Geometry check sheet. Reference: the model listing, model coordinates, mm. A direction names the side the tool comes from. Round coordinates to 2 decimals unless told otherwise and drop trailing zeros. Write each loop counter-clockwise with the first axis right and the second up, starting at its lowest first coordinate (ties: lowest second). Pieces come first, ordered by that corner, then holes. Notation, with made-up numbers: (-18.75, -27.5) -> (37.25, -27.5) arc R27 cw to (37.25, -10.5) -> close; hole circle Ø2 at (61, -2.5). An arc over 180 degrees is marked (long way). Return JSON: item names as keys, results as strings. Group by question number.
from build123d import *


with BuildPart() as f1:
    # F0 (on Front) → F1 (revolve)
    with BuildSketch(Plane.XZ):
        Polygon((0, -62), (0, 0), (-8, 0), (-8, -3.5), (-6, -3.5), (-6, -9.3), (-8, -9.3), (-8, -12.3), (-5.087018, -12.3), (-5.087018, -47.38391), (-6.285568, -47.38391), (-6.285568, -47.808396), (-5.087018, -47.808396), (-5.087018, -48.432641), (-9.75637, -48.432641), (-9.75637, -49.056886), (-5.087018, -49.056886), (-5.087018, -49.731071), (-9.75637, -49.731071), (-9.75637, -50.480166), (-5.087018, -50.480166), (-5.087018, -62), align=None)
    revolve(axis=Axis((0, 0, -31), (0, 0, 1)))


solid = f1.part
1) Go/stop test with flat-tipped pins: P1, Ø8, axis at y = 5.5, z = -50.5, coming from the +X side; P2, Ø1.5, axis at y = 1, z = -22.5, coming from the +X side; P3, Ø3, axis at x = -7.5, z = -12.5, coming from the -Y side. Record where each tip stops, or that it passes through.
2) Sectioned sample at A-A on z = -53.5. Enter the section's corners in (x, y).
3) Material ranges on probe 1 along Z at (x, y) = (-2.75, -5); probe 2 along Z at (x, y) = (-5.75, 3.75); probe 3 along Z at (x, y) = (4, -8.25), recorded low to high. Write a range as [from, to].
4) Tool access check on faces 1 (the face through (0.662, -5.044, -30.088)), 2 (the face through (1.73, 7.81, -1.77)), 3 (the face through (0.662, -5.044, -56.321)). Record the directions out of +Z, -Z, +X, -X, +Y, -Y that give a thin tool (end or side, any length) a straight path to the whole face; none if there is none.
5) Mould release check, pull along Z, two halves, no side actions. Record for faces 4 (the face through (-2, 5, -47.808)), 5 (the face through (1.27, -9.673, -48.749)), 6 (the face through (-4, 4, -50.48)), 7 (the face through (2, -6, -3.5)): +Z half, -Z half, draft (parallel to the pull), parting line (faces both ways), or undercut.
Evaluation:
{
 "1": {"P1": "stops at x = 9.64", "P2": "stops at x = 5.08", "P3": "stops at y = -5.28"},
 "2": {"outline": "circle Ø10.17 at (0, 0)"},
 "3": {"probe 1": "z = [-50.48, -49.73], [-49.06, -48.43], [-47.81, -47.38], [-12.3, 0]", "probe 2": "z = [-50.48, -49.73], [-49.06, -48.43], [-12.3, -9.3], [-3.5, 0]", "probe 3": "z = [-50.48, -49.73], [-49.06, -48.43]"},
 "4": {"face 1": "none", "face 2": "+Z", "face 3": "-Z"},
 "5": {"face 4": "undercut", "face 5": "draft", "face 6": "-Z half", "face 7": "undercut"}
}
